Geometry: final body of the model. Coordinates: model frame, mm. Face numbers are marked on the shaded views. A direction names the side the tool comes from. Round coordinates to 2 decimals unless told otherwise and drop trailing zeros. Loops run counter-clockwise (first coordinate to the right, second up) from the corner with the lowest first, then second, coordinate; pieces in that order, holes last. Notation, with made-up numbers: M -12.5,64 L -7.5,64 A12 ccw -7.5,83 Z; hole C -11,20 d10. An arc over 180 degrees is marked long. Return JSON: item names as keys, results as strings.
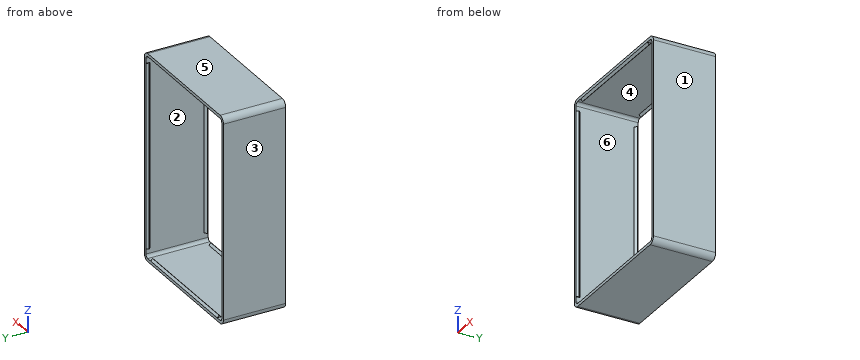
from build123d import *

# Parameters (mm, degrees)
SKETCH1_W           = 69.96
SKETCH1_H           = 102.98
SKETCH1_W_2         = 66.96
SKETCH1_H_2         = 99.98
BOSS_EXTRUDE1_DEPTH = 31.0002
FILLET1_R           = 3
FILLET2_R           = 1.5
BOSS_EXTRUDE2_START = -29.3587
BOSS_EXTRUDE2_DEPTH = 58.7174
BOSS_EXTRUDE3_START = -45.8687
BOSS_EXTRUDE3_DEPTH = 91.7374


with BuildPart() as part:
    # Sketch1 → Boss-Extrude1 (new body)
    with BuildSketch(Plane(origin=(0, 0, 0), x_dir=(1, 0, 0), z_dir=(0, 1, 0))):
        Rectangle(SKETCH1_W, SKETCH1_H)
        Rectangle(SKETCH1_W_2, SKETCH1_H_2, mode=Mode.SUBTRACT)
    extrude(amount=BOSS_EXTRUDE1_DEPTH)

    # Fillet1
    fillet1_edges = [part.edges().sort_by_distance(p)[0] for p in [
        (34.98, 15.5001, 51.49),
        (-34.98, 15.5001, 51.49),
        (-34.98, 15.5001, -51.49),
        (34.98, 15.5001, -51.49),
    ]]
    fillet(fillet1_edges, radius=FILLET1_R)

    # Fillet2
    fillet2_edges = [part.edges().sort_by_distance(p)[0] for p in [
        (-33.48, 15.5001, -49.99),
        (-33.48, 15.5001, 49.99),
        (33.48, 15.5001, 49.99),
        (33.48, 15.5001, -49.99),
    ]]
    fillet(fillet2_edges, radius=FILLET2_R)

    # Sketch2 → Boss-Extrude2 (add)
    with BuildSketch(Plane(origin=(0, 0, 0), x_dir=(0, 0, -1), z_dir=(1, 0, 0)).offset(BOSS_EXTRUDE2_START)):
        Polygon((-49.99, 31.0002), (-49.99, 29.0001972), (-48.9899986, 30.0001986), align=None)
        Polygon((49.99, 31.0002), (49.99, 29.0001972), (48.9899986, 30.0001986), align=None)
        Polygon((-49.99, 0), (-49.99, 2), (-48.99, 1), align=None)
        Polygon((49.99, 0), (49.99, 2), (48.99, 1), align=None)
    extrude(amount=BOSS_EXTRUDE2_DEPTH)

    # Sketch3 → Boss-Extrude3 (add)
    with BuildSketch(Plane.XY.offset(BOSS_EXTRUDE3_START)):
        Polygon((-33.48, 31.0002), (-33.48, 29.0001972), (-32.4799986, 30.0001986), align=None)
        Polygon((-33.48, 0), (-33.48, 2), (-32.48, 1), align=None)
        Polygon((33.48, 31.0002), (33.48, 29.0001972), (32.4799986, 30.0001986), align=None)
        Polygon((33.48, 0), (33.48, 2), (32.48, 1), align=None)
    extrude(amount=BOSS_EXTRUDE3_DEPTH)


solid = part.part
Q1. Reachability of the marked faces 1 and 2 from +Z, -Z, +X, -X, +Y, -Y: full face, straight path, thin tool, end or side. Return the list, or none.
Determined:
{"face 1": "+Z, -Z, +X, +Y, -Y", "face 2": "none"}
Q2. Section query B-B (y = 16.5). Output: boundary loops of the cut face in (x, z), plus the area to 3 significant figures.
Determined:
{"outline": "M -34.98,-48.49 A3 ccw -31.98,-51.49 L 31.98,-51.49 A3 ccw 34.98,-48.49 L 34.98,48.49 A3 ccw 31.98,51.49 L -31.98,51.49 A3 ccw -34.98,48.49 Z; hole M -33.48,-48.49 A1.5 ccw -31.98,-49.99 L 31.98,-49.99 A1.5 ccw 33.48,-48.49 L 33.48,48.49 A1.5 ccw 31.98,49.99 L -31.98,49.99 A1.5 ccw -33.48,48.49 Z", "area": "504 mm^2"}
Q3. Section query C-C (x = -2). Output: boundary loops of the cut face in (y, z), plus the area to 3 significant figures.
Determined:
{"outline": "M 0,-51.49 L 31,-51.49 L 31,-49.99 L 30,-48.99 L 29,-49.99 L 2,-49.99 L 1,-48.99 L 0,-49.99 Z; M 0,49.99 L 1,48.99 L 2,49.99 L 29,49.99 L 30,48.99 L 31,49.99 L 31,51.49 L 0,51.49 Z", "area": "97.0 mm^2"}
Q4. Material intervals for L1, parallel to Z at x = 19, y = 25; L2, parallel to X at y = 17, z = 19, sorted ascending.
Determined:
{"L1": "z = -51.49 to -49.99, 49.99 to 51.49", "L2": "x = -34.98 to -33.48, 33.48 to 34.98"}
Q5. Section query A-A (z = 6). Output: boundary loops of the cut face in (x, y), plus the area to 3 significant figures.
Determined:
{"outline": "M -34.98,0 L -33.48,0 L -32.48,1 L -33.48,2 L -33.48,29 L -32.48,30 L -33.48,31 L -34.98,31 Z; M 32.48,1 L 33.48,0 L 34.98,0 L 34.98,31 L 33.48,31 L 32.48,30 L 33.48,29 L 33.48,2 Z", "area": "97.0 mm^2"}
Q6. Pin query (flat end, axial travel): pin 1 (0.5 mm diameter, centred on y = 0.5, z = -49.5, fed in from +X); pin 2 (0.5 mm diameter, centred on x = -33, y = 1, fed in from +Z); pin 3 (0.8 mm diameter, centred on x = 33, y = 1, fed in from -Z). Return the tip coordinate at first contact, or that it passes through.
Determined:
{"pin 1": "stops at x = 34.88", "pin 2": "stops at z = 51.39", "pin 3": "stops at z = -51.43"}
Q7. Pull-direction query (Z, two-part tool) for the marked faces 3, 4, 5 and 6; classes: pulls with the +Z half, pulls with the -Z half, needs draft (parallel to the pull), parting line crosses it, or undercut.
Determined:
{"face 3": "needs draft", "face 4": "undercut", "face 5": "pulls with the +Z half", "face 6": "undercut"}
